Autodesk Inventor part; units mm, degrees
ref_plane "Work Plane1" through (22.5184, 2.463, -18.3509) normal (0, 0, 1) x (0.9997722, -0.0213418, 0)
ref_plane "YZ Plane" through (0, 0, 0) normal (1, 0, 0) x (0, 1, 0)
ref_plane "XZ Plane" through (0, 0, 0) normal (0, 1, 0) x (-1, 0, 0)
ref_plane "Work Plane1" through (22.5184, 2.463, -18.3509) normal (0, 0, 1) x (0.9997722, -0.0213418, 0)
sketch "ThermoBulbBorder" plane through (22.5184, 2.463, -18.3509) normal (0, 0, 1) x (0.9997722, -0.0213418, 0)
  arc A0 (-447.455, -468.958) -> (162.145, -468.958) centre (-142.655, -774.8145) ccw
  arc A1 (-447.455, -468.958) -> (162.145, -468.958) centre (-142.655, -774.8145) ccw
  arc A2 (-383.955, -588.5959) -> (98.645, -588.5959) centre (-142.655, -774.8145) ccw
  line L0 (-447.455, -468.958) -> (-383.955, -468.958)
  line L1 (-383.955, -468.958) -> (-383.955, -588.5959)
  line L2 (162.145, -468.958) -> (98.645, -468.958)
  line L3 (98.645, -468.958) -> (98.645, -588.5959)
  line L4 (-383.955, -961.033) -> (-484.4967, -1038.6241)
  line L5 (98.645, -961.033) -> (199.1867, -1038.6241)
  arc A3 (-447.455, -468.958) -> (162.145, -468.958) centre (-142.655, -774.8145) ccw
  circle A4 centre (-142.655, -774.8145) radius 419.1 construction
  circle A5 centre (-142.655, -774.8145) radius 406.908 construction
  circle A6 centre (-142.655, -774.8145) radius 349.758 construction
  circle A7 centre (-142.655, -774.8145) radius 337.566 construction
  line L6 (98.645, -468.958) -> (98.645, -316.558) construction
  line L7 (-383.955, -468.958) -> (-383.955, -316.558) construction
  dimension "d0" = 609.6
  dimension "d5" = 63.5
  dimension "d6" = 63.5
  dimension "d7" = 838.2
  dimension "d8" = 12.192
  dimension "d9" = 12.192
  dimension "d10" = 57.15
  dimension "d11" = 32.766
  dimension "d12" = 152.4
extrude "Extrusion2" add sketch "ThermoBulbBorder" along normal blind 18.034 contours L4 A2 L5 A0
sketch "Sketch2" plane through (22.5184, 2.463, -0.3169) normal (0, 0, 1) x (0.9997722, -0.0213418, 0)
  line L0 (-383.955, -961.033) -> (-484.4967, -1038.6241)
  arc A0 (-484.4967, -1038.6241) -> (199.1867, -1038.6241) centre (-142.655, -774.8145) ccw
  line L1 (199.1867, -1038.6241) -> (98.645, -961.033)
  arc A1 (-383.955, -961.033) -> (98.645, -961.033) centre (-142.655, -774.8145) ccw
  arc A2 (-409.8948, -981.0515) -> (124.5847, -981.0515) centre (-142.655, -774.8145) ccw
  arc A3 (-419.5468, -988.5003) -> (134.2367, -988.5003) centre (-142.655, -774.8145) ccw
  arc A4 (-464.7905, -1023.4163) -> (179.4805, -1023.4163) centre (-142.655, -774.8145) ccw
  arc A5 (-474.4425, -1030.865) -> (189.1325, -1030.865) centre (-142.655, -774.8145) ccw
  line L2 (-474.4425, -1030.865) -> (-464.7905, -1023.4163)
  line L3 (-419.5468, -988.5003) -> (-409.8948, -981.0515)
  line L4 (124.5847, -981.0515) -> (134.2367, -988.5003)
  line L5 (179.4805, -1023.4163) -> (189.1325, -1030.865)
  point P0 (-22.4607, -2.943)
  dimension "d15" = 12.192
  dimension "d17" = 12.7
  dimension "d18" = 57.15
  dimension "d19" = 12.192
extrude "Extrusion3" cut sketch "Sketch2" against normal blind 12.7 contours A2 L1 A3 L0 | A4 L1 A5 L0
equation "\"d6\" = d5"
equation "\"d8\" = bRopeChannel"
equation "\"d9\" = bRopeChannel"
equation "\"d15\" = bRopeChannel"
equation "\"d19\" = bRopeChannel"
equation "\"bRopeChannel\" = 12.192"
properties part number "HOT Thermo bulb outline B" material "Rubber, Butyl"
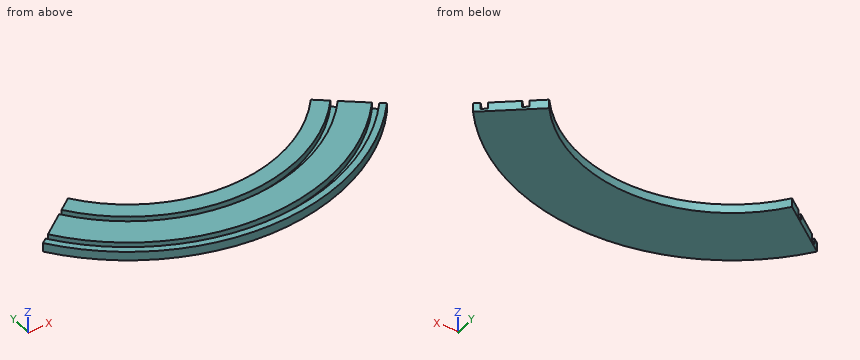
Verification items for the finished model (mm, model axes). Coordinates: 2 decimals unless noted, no trailing zeros. Order: outer loops, then holes, each group sorted by start corner. A loop starts at its lowest first (then second) coordinate and runs counter-clockwise, first axis right, second up. Notation, with made-up numbers: M -27.5,7.25 L -4.5,7.25 A23 cw -4.5,17.25 Z; hole C 42.5,-16 d9. An arc over 180 degrees is marked long. One line per item, written item: value. Start each with the question number.
Item 1: Depth check by flat-ended pin: P1, Ø2, axis at y = -1111, z = -9, coming from the -X side; P2, Ø4, axis at x = -249.5, y = -1096.5, coming from the +Z side; P3, Ø5, axis at y = -1118.5, z = -8, coming from the -X side. Enter the tip coordinate at first touch or a pass-through.
Item 2: Sectioned sample at C-C on y = -1140. Record the cut outline in (x, z), then the cut area to 3 significant figures.
Item 3: Sectioned sample at B-B on x = -8. Record the cut outline in (y, z).
Item 4: Thickness scan on probe 1 along Y at (x, z) = (-104.5, -11.75); probe 2 along Y at (x, z) = (-324, -12.5); probe 3 along X at (y, z) = (-1051, -6.5). Record the ranges inside material, lowest first.
Item 5: Sectioned sample at A-A on z = -3.5. Record the cut outline in (x, y), then the cut area to 3 significant figures.
Calculated:
1. P1: x = -401.7
1. P2: z = -13.02
1. P3: x = -393.8
2. outline: M -357.79,-18.35 L 84.51,-18.35 L 84.51,-0.32 L 58.55,-0.32 L 58.55,-13.02 L 30.78,-13.02 L 30.78,-0.32 L -304.06,-0.32 L -304.06,-13.02 L -331.83,-13.02 L -331.83,-0.32 L -357.79,-0.32 Z
2. area: 7,270 mm^2
3. outline: M -1181.32,-18.35 L -1045.45,-18.35 L -1045.45,-0.32 L -1081.22,-0.32 L -1081.22,-13.02 L -1094.37,-13.02 L -1094.37,-0.32 L -1155.17,-0.32 L -1155.17,-13.02 L -1168,-13.02 L -1168,-0.32 L -1181.32,-0.32 Z
4. probe 1: -1199.73 to -1187, -1174.77 to -1117.41, -1105.16 to -1072.23
4. probe 2: -1158.16 to -1144.02, -1130.34 to -1064.47, -1049.93 to -1009.55
4. probe 3: -463.75 to -446.79, -430.11 to -343.72, -322.38 to -252.63, -20.65 to 49.1, 70.44 to 156.83, 173.51 to 190.47
5. outline: M -484.03,-1025.58 A431.8 ccw 199.49,-1040.18 L 189.61,-1032.2 A419.1 cw -473.82,-1018.04 Z; M -464.01,-1010.8 A406.91 ccw 180.12,-1024.55 L 135.63,-988.68 A349.76 cw -418.03,-976.86 Z; M -408.22,-969.62 A337.57 ccw 126.14,-981.02 L 100.63,-960.46 A304.8 cw -381.86,-950.16 Z
5. area: 68,600 mm^2
